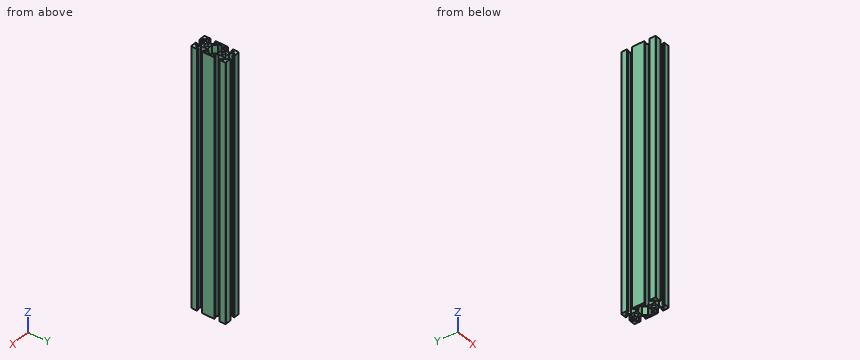
from build123d import *

# Parameters (mm, degrees)
SCHIZZO1_R                   = 2.1
ESTRUSIONE_ESTRUSIONE1_DEPTH = 300
RACCORDO1_R                  = 1


with BuildPart() as part:
    # Schizzo1 → Estrusione-Estrusione1 (new body)
    with BuildSketch(Plane.XY):
        Polygon((-3, 20), (-10, 20), (-10, 13), (-8, 13), (-8, 16), (-7, 16), (-4, 13), (-4, 7), (-7, 4), (-8, 4), (-8, 7), (-10, 7), (-10, -7), (-8, -7), (-8, -4), (-7, -4), (-4, -7), (-4, -13), (-7, -16), (-8, -16), (-8, -13), (-10, -13), (-10, -20), (-3, -20), (-3, -18), (-6, -18), (-6, -17), (-3, -14), (3, -14), (6, -17), (6, -18), (3, -18), (3, -20), (10, -20), (10, -13), (8, -13), (8, -16), (7, -16), (4, -13), (4, -7), (7, -4), (8, -4), (8, -7), (10, -7), (10, 7), (8, 7), (8, 4), (7, 4), (4, 7), (4, 13), (7, 16), (8, 16), (8, 13), (10, 13), (10, 20), (3, 20), (3, 18), (6, 18), (6, 17), (3, 14), (-3, 14), (-6, 17), (-6, 18), (-3, 18), align=None)
        Polygon((8, 2), (8, -2), (7, -2), (3, -6), (-3, -6), (-7, -2), (-8, -2), (-8, 2), (-7, 2), (-3, 6), (3, 6), (7, 2), align=None, mode=Mode.SUBTRACT)
        with Locations((0, 10)):
            Circle(SCHIZZO1_R, mode=Mode.SUBTRACT)
        with Locations((0, -10)):
            Circle(SCHIZZO1_R, mode=Mode.SUBTRACT)
    extrude(amount=ESTRUSIONE_ESTRUSIONE1_DEPTH)

    # Raccordo1
    raccordo1_edges = [part.edges().sort_by_distance(p)[0] for p in [
        (-10, 20, 150),
        (10, 20, 150),
        (10, -20, 150),
        (-10, -20, 150),
    ]]
    fillet(raccordo1_edges, radius=RACCORDO1_R)


solid = part.part
Work out the finished part from the listing and answer in its coordinate system (mm). Coordinates: 2 decimals unless noted, no trailing zeros. Write item = value, one per line.
1. The part is cut by section A-A (z = 29). State how many separate pieces and enclosed holes the cut face has, then the cut area to 3 significant figures.
Solution:
separate_pieces = 1
enclosed_holes = 3
area = 321 mm2
2. Flat-ended cylindrical pins translate along their axes: pin 1 (6.5 mm diameter, centred on x = -0.5, z = 96.5, fed in from -Y); pin 2 (1.8 mm diameter, centred on y = -9, z = 158.5, fed in from +X). Find the tip coordinate at first contact, or state that the pin passes through.
Solution:
pin_1 = -20
pin_2 = 4
3. Straight lines are drawn through the part: line 1 (Y direction, x = 0, z = 177); line 2 (Y direction, x = -7, z = 47); line 3 (X direction, y = -5, z = 235). For each, find the intervals that lie inside material, in ascending order. Write a range as from..to.
Solution:
line_1 = -14..-12.1, -7.9..-6, 6..7.9, 12.1..14
line_2 = -20..-16, -4..-2, 2..4, 16..20
line_3 = -10..-8, -6..-4, 4..6, 8..10
